Verification items for the finished model (mm, model axes). A direction names the side the tool comes from. Round coordinates to 2 decimals unless told otherwise and drop trailing zeros. Write each loop counter-clockwise with the first axis right and the second up, starting at its lowest first coordinate (ties: lowest second). Pieces come first, ordered by that corner, then holes. Notation, with made-up numbers: (-1.75, -38.75) -> (2.25, -38.75) arc R13 ccw to (2.25, -31.75) -> close; hole circle Ø5 at (-30.5, 43). An arc over 180 degrees is marked (long way). Answer as a JSON object with one key per item and string values. Group by question number.
(1) Gauge pin test, flat ends, axial feed: pin 1 Ø4 at (x, z) = (11, -8) entering from -Y; pin 2 Ø3 at (x, z) = (40.5, 5.5) entering from +Y; pin 3 Ø2 at (x, z) = (18.5, 2.5) entering from -Y. Record the tip position at first contact, or that the pin passes through.
(2) Set-up check for faces 1 (the face through (51, -10, -5)), 2 (the face through (25.14, -10.74, 2.38)): record each of +Z, -Z, +X, -X, +Y, -Y from which the full face is reachable in a straight line by a thin tool's end or side.
(3) Sectioned sample at C-C on x = 8. Record the cut outline in (y, z).
(4) Scan lines: L1, parallel to Y at x = 40, z = -0.25; L2, parallel to Z at x = 1.5, y = -10; L3, parallel to X at y = -7, z = -3.5. Record each from-to range of solid material in increasing order. Write a range as from..to.
(5) Sectioned sample at A-A on y = 0. Record the cut outline in (x, z), and give its area (3 significant figures).
(6) Draft check along Y on faces 3 (the face through (0, 0, 0)), 4 (the face through (-6, 0, 0)), 5 (the face through (22.101, 3.755, -11.923)). Enter one of: released by +Y, released by -Y, zero draft, split by the parting line, or undercut.
```python
from build123d import *

# Parameters (mm, degrees)
CYLINDER006_R           = 11
CYLINDER006_DEPTH       = 51
CYLINDER006_PITCH_ANGLE = 90
CYLINDER005_R           = 12.5
CYLINDER005_DEPTH       = 57
CYLINDER005_PITCH_ANGLE = 90


with BuildPart() as cylinder004:
    # Cylinder006 → Cylinder006 (new body)
    with BuildSketch(Plane.XY):
        Circle(CYLINDER006_R)
    extrude(amount=CYLINDER006_DEPTH)


with BuildPart() as cylinder004_1:
    # Cylinder006 pitch: moved
    add(cylinder004.part.rotate(Axis((0, 0, 0), (0, 1, 0)), CYLINDER006_PITCH_ANGLE))


with BuildPart() as cylinder004_2:
    # Cylinder006 placement: moved
    add(cylinder004_1.part)


with BuildPart() as batterycap:
    # Cylinder005 → Cylinder005 (new body)
    with BuildSketch(Plane.XY):
        Circle(CYLINDER005_R)
    extrude(amount=CYLINDER005_DEPTH)


with BuildPart() as batterycap_1:
    # Cylinder005 pitch: moved
    add(batterycap.part.rotate(Axis((0, 0, 0), (0, 1, 0)), CYLINDER005_PITCH_ANGLE))


with BuildPart() as batterycap_2:
    # Cylinder005 placement: moved
    add(batterycap_1.part.moved(Location((-6, 0, 0))))

    # Cut003: cut Cylinder004
    add(cylinder004_2.part, mode=Mode.SUBTRACT)


solid = batterycap_2.part
```
Computed values:
{
 "1": {"pin 1": "y = -10.97", "pin 2": "y = 11.84", "pin 3": "y = -12.41"},
 "2": {"face 1": "+Z, -Z, +X, +Y, -Y", "face 2": "+X"},
 "3": {"outline": "circle Ø25 at (0, 0); hole circle Ø22 at (0, 0)"},
 "4": {"L1": "-12.5..-11, 11..12.5", "L2": "-7.5..-4.58, 4.58..7.5", "L3": "-6..0"},
 "5": {"outline": "(-6, -12.5) -> (51, -12.5) -> (51, -11) -> (0, -11) -> (0, 11) -> (51, 11) -> (51, 12.5) -> (-6, 12.5) -> close", "area": "303 mm2"},
 "6": {"face 3": "undercut", "face 4": "zero draft", "face 5": "split by the parting line"}
}
